Could you check a few things on this model? Use its own coordinates, in mm. A direction names the side the tool comes from. Give positions to 0.01 mm unless a question says otherwise; leave off trailing zeros. Loops run counter-clockwise (first coordinate to the right, second up) from the corner with the lowest first, then second, coordinate; pieces in that order, holes last. Notation, with made-up numbers: M -15,9 L 18,9 A16 ccw 18,19 Z; hole C 8,68 d6. An arc over 180 degrees is marked long. Use a Markdown table: item, result. Add a question column.
1) Suppose I cut it at A-A on x = 5. List the corners of the cut face in (y, z) for me.
2) Which directions (+Z, -Z, +X, -X, +Y, -Y) give clear straight access to the entire face, cutting with the end or side of a thin tool? Please do faces 4 (the flat face through (-1.392, -4.93, 3.116)), 5 (the flat face through (3.116, -4.93, 1.392)), 6 (the flat face through (-1.76, -4.93, 1.77)), 7 (the flat face through (1.388, -4.93, 3.093)).
3) If I drill on line 1 along Z through (x, y) = (0, -4); line 2 along X through (y, z) = (-1, 6.75); line 3 along X through (y, z) = (-1, 0.75), over which ranges is the centre line in solid material (lowest first)? Write a range as [from, to].
4) We'd pull the mould along X, two halves only. Please class faces 1 (the flat face through (1.836, -4.93, 5.234)), 2 (the flat face through (-3.093, -4.93, 1.388)), 3 (the flat face through (-6.793, -4.93, 0.971)): +X half, -X half, draft (parallel to the pull), parting line (faces both ways), or undercut.
5) Will these pins go through, and if not, where does the flat tip stop? pin 1 Ø4 at (x, y) = (2.5, -3) entering from -Z; pin 2 Ø1 at (y, z) = (-6, -6) entering from +X.
6) Suppose I cut it at B-B on z = -3.5. List the corners of the cut face in (x, y) for me.
```python
from build123d import *

# Parameters (mm, degrees)
F1_DEPTH = 10


with BuildPart() as f1:
    # F0 (on Front) → F1 (new body)
    with BuildSketch(Plane.XZ):
        Polygon((-1.680939, -5.992074), (-0.241203, -7.615681), (0, -7.639437), (0.241203, -7.615681), (1.680939, -5.992074), (1.986931, -4.496766), (1.908474, -4.261395), (1.532129, -3.927671), (1.248645, -2.281909), (2.281909, -1.248645), (3.927671, -1.532129), (4.261395, -1.908474), (4.496766, -1.986931), (5.992074, -1.680939), (7.615681, -0.241203), (7.639437, 0), (7.615681, 0.241203), (5.992074, 1.680939), (4.496766, 1.986931), (4.261395, 1.908474), (3.927671, 1.532129), (2.281909, 1.248645), (1.248645, 2.281909), (1.532129, 3.927671), (1.908474, 4.261395), (1.986931, 4.496766), (1.680939, 5.992074), (0.241203, 7.615681), (0, 7.639437), (-0.241203, 7.615681), (-1.680939, 5.992074), (-1.986931, 4.496766), (-1.908474, 4.261395), (-1.532129, 3.927671), (-1.248645, 2.281909), (-2.281909, 1.248645), (-3.927671, 1.532129), (-4.261395, 1.908474), (-4.496766, 1.986931), (-5.992074, 1.680939), (-7.615681, 0.241203), (-7.639437, 0), (-7.615681, -0.241203), (-5.992074, -1.680939), (-4.496766, -1.986931), (-4.261395, -1.908474), (-3.927671, -1.532129), (-2.281909, -1.248645), (-1.248645, -2.281909), (-1.532129, -3.927671), (-1.908474, -4.261395), (-1.986931, -4.496766), align=None)
        Polygon((0.44741, -1.0049), (0.228703, -1.075962), (0, -1.1), (-0.228703, -1.075962), (-0.44741, -1.0049), (-0.646564, -0.889919), (-0.817459, -0.736044), (-0.952628, -0.55), (-1.046162, -0.339919), (-1.093974, -0.114981), (-1.093974, 0.114981), (-1.046162, 0.339919), (-0.952628, 0.55), (-0.817459, 0.736044), (-0.646564, 0.889919), (-0.44741, 1.0049), (-0.228703, 1.075962), (0, 1.1), (0.228703, 1.075962), (0.44741, 1.0049), (0.646564, 0.889919), (0.817459, 0.736044), (0.952628, 0.55), (1.046162, 0.339919), (1.093974, 0.114981), (1.093974, -0.114981), (1.046162, -0.339919), (0.952628, -0.55), (0.817459, -0.736044), (0.646564, -0.889919), align=None, mode=Mode.SUBTRACT)
    extrude(amount=F1_DEPTH)


solid = f1.part
```
Answer block:
| question | item | result |
|---|---|---|
| 1 | outline | M -10,-1.88 L 0,-1.88 L 0,1.88 L -10,1.88 Z |
| 2 | face 4 | -X, +Y, -Y |
| 2 | face 5 | +Z, +Y, -Y |
| 2 | face 6 | +Y, -Y |
| 2 | face 7 | +X, +Y, -Y |
| 3 | line 1 | z = [-7.64, -1.1], [1.1, 7.64] |
| 3 | line 2 | x = [-1.01, 1.01] |
| 3 | line 3 | x = [-7.04, -0.8], [0.8, 7.04] |
| 4 | face 1 | +X half |
| 4 | face 2 | undercut |
| 4 | face 3 | -X half |
| 5 | pin 1 | stops at z = -7.32 |
| 5 | pin 2 | stops at x = 1.78 |
| 6 | outline | M -1.46,-10 L 1.46,-10 L 1.46,0 L -1.46,0 Z |
